Work out the finished part from the listing and answer in its coordinate system (mm). A direction names the side the tool comes from. Round coordinates to 2 decimals unless told otherwise and drop trailing zeros. Loops run counter-clockwise (first coordinate to the right, second up) from the corner with the lowest first, then second, coordinate; pieces in that order, holes last. Notation, with made-up numbers: (86.25, -23) - (142.25, -23) arc R8 cw to (142.25, -9) - close; hole circle Ø3 at (5.25, -15). An arc over 180 degrees is marked (long way). Return JSON: item names as keys, results as strings.
from build123d import *
from build123d.topology import SkipClean

# Parameters (mm, degrees)
SKETCH1_R           = 9.906
BOSS_EXTRUDE1_DEPTH = 6.35
FILLET1_START       = -3.8100001
FILLET1_3_DEPTH     = 3.8100001
FILLET2_R           = 1.27


with BuildPart() as part:
    # Sketch1 → Boss-Extrude1 (new body)
    with BuildSketch(Plane.XY):
        with BuildLine():
            ThreePointArc((-9.873287403, 0.804382899), (-9.42116585, 3.061122346), (-8.460461705, 5.152613292))
            Line((-8.460461705, 5.152613292), (-10.513792724, 5.819780983))
            ThreePointArc((-10.513792724, 5.819780983), (-13.394320769, 4.352078636), (-11.926618422, 1.47155059))
            Line((-11.926618422, 1.47155059), (-9.873287403, 0.804382899))
        make_face()
        Circle(SKETCH1_R)
        with BuildLine():
            Line((-5.085055556, -10.888154027), (-3.816027196, -9.141486336))
            ThreePointArc((-3.816027196, -9.141486336), (-5.822600709, -8.014122346), (-7.514852894, -6.454132163))
            Line((-7.514852894, -6.454132163), (-8.783881254, -8.200799854))
            ThreePointArc((-8.783881254, -8.200799854), (-8.278145492, -11.39388979), (-5.085055556, -10.888154027))
        make_face()
        with BuildLine():
            Line((8.783881254, -8.200799854), (7.514852894, -6.454132163))
            ThreePointArc((7.514852894, -6.454132163), (5.822600709, -8.014122346), (3.816027196, -9.141486336))
            Line((3.816027196, -9.141486336), (5.085055556, -10.888154027))
            ThreePointArc((5.085055556, -10.888154027), (8.278145492, -11.39388979), (8.783881254, -8.200799854))
        make_face()
        with BuildLine():
            Line((9.873287403, 0.804382899), (11.926618422, 1.47155059))
            ThreePointArc((11.926618422, 1.47155059), (13.394320769, 4.352078636), (10.513792724, 5.819780983))
            Line((10.513792724, 5.819780983), (8.460461705, 5.152613292))
            ThreePointArc((8.460461705, 5.152613292), (9.42116585, 3.061122346), (9.873287403, 0.804382899))
        make_face()
        with BuildLine():
            ThreePointArc((-2.286, 9.638622308), (0, 9.906), (2.286, 9.638622308))
            Line((2.286, 9.638622308), (2.286, 11.797622308))
            ThreePointArc((2.286, 11.797622308), (0, 14.083622308), (-2.286, 11.797622308))
            Line((-2.286, 11.797622308), (-2.286, 9.638622308))
        make_face()
    extrude(amount=BOSS_EXTRUDE1_DEPTH)

    # Sketch2 → Revolve1 (revolve)
    with SkipClean():  # the faces are left unmerged after this step: merging them gives an invalid solid
        with BuildSketch(Plane(origin=(0, 0, 0), x_dir=(1, 0, 0), z_dir=(0, 1, 0))):
            Polygon((0, 50.8), (0, 0), (9.906, 0), (9.906, 5.08), (6.35, 8.636), (6.35, 39.37), (12.7, 45.72), (12.7, 50.8), align=None)
        revolve(axis=Axis((0, 0, 0), (0, 0, -1)))
    add(part.part.scale(1), mode=Mode.REPLACE)  # the faces are merged on a copy

    # Fillet1: read off the stored shape, not the designer's step
    # Fillet1 outline → Fillet1 (revolve, cut)
    with BuildSketch(Plane.XZ):
        with BuildLine():
            Line((12.7, -44.604076836), (11.584076836, -44.604076836))
            ThreePointArc((11.584076836, -44.604076836), (12.409981019, -45.840129795), (12.7, -47.298153673))
            Line((12.7, -47.298153673), (12.7, -44.604076836))
        make_face()
    revolve(axis=Axis((0, 0, 0), (0, 0, 1)), mode=Mode.SUBTRACT)

    # Fillet1 2 outline → Fillet1 2 (revolve)
    with BuildSketch(Plane.XZ):
        with BuildLine():
            Line((6.35, -40.485923164), (7.465923164, -40.485923164))
            ThreePointArc((7.465923164, -40.485923164), (6.640018981, -39.249870205), (6.35, -37.791846327))
            Line((6.35, -37.791846327), (6.35, -40.485923164))
        make_face()
        with BuildLine():
            Line((6.35, -7.520076836), (6.35, -10.214153673))
            ThreePointArc((6.35, -10.214153673), (6.640018981, -8.756129795), (7.465923164, -7.520076836))
            Line((7.465923164, -7.520076836), (6.35, -7.520076836))
        make_face()
    revolve(axis=Axis((0, 0, 0), (0, 0, 1)))

    # Fillet1 3 outline → Fillet1 3 (add)
    with BuildSketch(Plane.XY.offset(FILLET1_START)):
        with BuildLine():
            Line((-11.926618422, 1.47155059), (-9.873287403, 0.804382899))
            ThreePointArc((-9.873287403, 0.804382899), (-9.42116585, 3.061122346), (-8.460461705, 5.152613292))
            Line((-8.460461705, 5.152613292), (-10.513792724, 5.819780983))
            ThreePointArc((-10.513792724, 5.819780983), (-13.394320769, 4.352078635), (-11.926618422, 1.47155059))
        make_face()
        with BuildLine():
            ThreePointArc((-3.816027196, -9.141486336), (-5.822600709, -8.014122346), (-7.514852894, -6.454132163))
            Line((-7.514852894, -6.454132163), (-8.783881254, -8.200799854))
            ThreePointArc((-8.783881254, -8.200799854), (-8.278145492, -11.39388979), (-5.085055556, -10.888154027))
            Line((-5.085055556, -10.888154027), (-3.816027196, -9.141486336))
        make_face()
        with BuildLine():
            Line((-2.286, 11.797622308), (-2.286, 9.638622308))
            ThreePointArc((-2.286, 9.638622308), (0, 9.906), (2.286, 9.638622308))
            Line((2.286, 9.638622308), (2.286, 11.797622308))
            ThreePointArc((2.286, 11.797622308), (0, 14.083622308), (-2.286, 11.797622308))
        make_face()
        with BuildLine():
            ThreePointArc((7.514852894, -6.454132163), (5.822600709, -8.014122346), (3.816027196, -9.141486336))
            Line((3.816027196, -9.141486336), (5.085055556, -10.888154027))
            ThreePointArc((5.085055556, -10.888154027), (8.278145492, -11.39388979), (8.783881254, -8.200799854))
            Line((8.783881254, -8.200799854), (7.514852894, -6.454132163))
        make_face()
        with BuildLine():
            Line((10.513792724, 5.819780983), (8.460461705, 5.152613292))
            ThreePointArc((8.460461705, 5.152613292), (9.42116585, 3.061122346), (9.873287403, 0.804382899))
            Line((9.873287403, 0.804382899), (11.926618422, 1.47155059))
            ThreePointArc((11.926618422, 1.47155059), (13.394320769, 4.352078635), (10.513792724, 5.819780983))
        make_face()
    extrude(amount=FILLET1_3_DEPTH)

    # Fillet1 4 outline → Fillet1 4 (revolve, cut)
    with BuildSketch(Plane.XZ):
        with BuildLine():
            Line((14.083622308, 0), (13.716, 0))
            ThreePointArc((13.716, 0), (11.021923164, -1.115923164), (9.906, -3.81))
            Line((9.906, -3.81), (14.083622308, -3.8100001))
            Line((14.083622308, -3.8100001), (14.083622308, 0))
        make_face()
    revolve(axis=Axis((0, 0, 0), (0, 0, 1)), mode=Mode.SUBTRACT)

    # Fillet2
    fillet2_edges = [part.edges().sort_by_distance(p)[0] for p in [
        (-12.7, 0, -50.8),
    ]]
    fillet(fillet2_edges, radius=FILLET2_R)


solid = part.part
1) Flat-ended cylindrical pins translate along their axes: pin 1 (0.5 mm diameter, centred on x = -13, y = 4, fed in from -Z); pin 2 (10 mm diameter, centred on y = 7, z = -10, fed in from +X); pin 3 (1.1 mm diameter, centred on y = 10.5, z = 2, fed in from +X). Find the tip coordinate at first contact, or state that the pin passes through.
Verdict:
{"pin 1": "stops at z = -0.02", "pin 2": "stops at x = 8.17", "pin 3": "stops at x = 2.29"}
2) Determine the mould class of faces 1 (the flat face through (0, 1, 6.35)), 2 (the flat face through (8.2, -11.2, 0)), 3 (the flat face through (-10.91, 1.14, 2.33)), 4 (the conical face through (3.5, 6.73, -7.4)) for opening direction Z: pulls with the +Z half, pulls with the -Z half, needs draft (parallel to the pull), parting line crosses it, or undercut.
Verdict:
{"face 1": "pulls with the +Z half", "face 2": "pulls with the -Z half", "face 3": "needs draft", "face 4": "undercut"}
3) Section A-A (x = 0) is taken. Give the vertices of the cut face in (y, z), and give its area (3 significant figures).
Verdict:
{"outline": "(-12.7, -49.53) arc R1.27 ccw to (-11.43, -50.8) - (11.43, -50.8) arc R1.27 ccw to (12.7, -49.53) - (12.7, -47.3) arc R3.81 ccw to (11.58, -44.6) - (7.47, -40.49) arc R3.81 cw to (6.35, -37.79) - (6.35, -10.21) arc R3.81 cw to (7.47, -7.52) - (9.91, -5.08) - (9.91, -3.81) arc R3.81 cw to (13.72, 0) - (14.08, 0) - (14.08, 6.35) - (-9.91, 6.35) - (-9.91, -5.08) - (-7.47, -7.52) arc R3.81 cw to (-6.35, -10.21) - (-6.35, -37.79) arc R3.81 cw to (-7.47, -40.49) - (-11.58, -44.6) arc R3.81 ccw to (-12.7, -47.3) - close", "area": "954 mm2"}
4) Section B-B (z = -16.5) is taken. Give the vertices of the cut face in (x, y).
Verdict:
{"outline": "circle Ø12.7 at (0, 0)"}
5) Find the intervals of material crossed by L1, parallel to Z at x = -8.5, y = -11; L2, parallel to Z at x = 1.5, y = -7; L3, parallel to Z at x = -7.75, y = 0.25, in increasing order.
Verdict:
{"L1": "z = 0 to 6.35", "L2": "z = -50.8 to -40.14, -7.87 to 6.35", "L3": "z = -50.8 to -40.77, -7.23 to 6.35"}
6) A tool of negligible diameter and unlimited length cuts with its end or side. For faces 5 (the conical face through (7.367, -2.32, -40.744)), 6 (the cylindrical face through (-2.75, 12.4, -48.43)), 7 (the flat face through (-8.2, -11.2, 0)), 8 (the flat face through (0, 0, -50.8)), from which of +Z, -Z, +X, -X, +Y, -Y can it reach the whole face along a straight path? Write none if from no direction.
Verdict:
{"face 5": "none", "face 6": "-Z", "face 7": "-Z, -X, -Y", "face 8": "-Z, +X, -X, +Y, -Y"}
